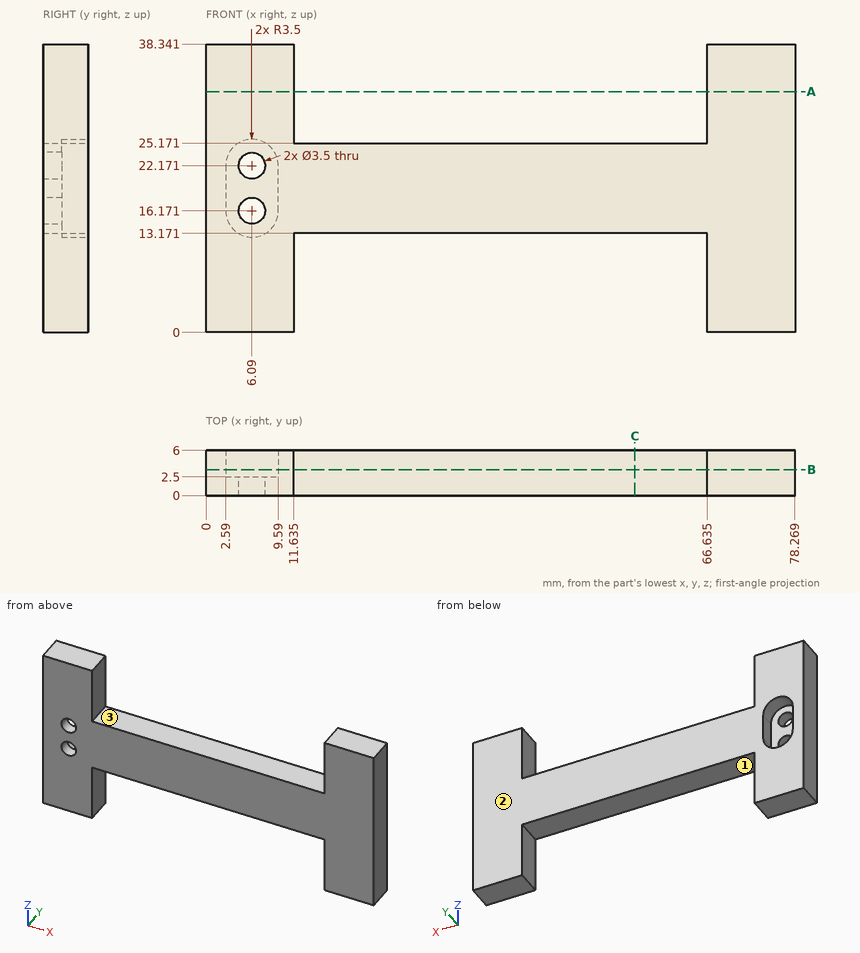
Print and shaded views of the part. All mm, measured from the part's lowest x, y and z. A direction names the side the tool comes from. Coordinates: 2 decimals unless noted, no trailing zeros. Order: outer loops, then holes, each group sorted by start corner. A loop starts at its lowest first (then second) coordinate and runs counter-clockwise, first axis right, second up. Notation, with made-up numbers: (74, -16) - (85, -16) arc R18 ccw to (85, 18) - close; hole circle Ø1 at (26, 29.25). An arc over 180 degrees is marked (long way). Return JSON: item names as keys, results as strings. Group by question number.
Item 1: Pin check, flat tips, straight feed: pin 1 (5.5 mm diameter, centred on x = 6.5, z = 17.5, fed in from +Y); pin 2 (3 mm diameter, centred on x = 45, y = 4.5, fed in from -Z). Stop position of each tip, or through.
Item 2: Cut at C-C (x = 57). List the corners of the cut face in (y, z), plus the area to 3 significant figures.
Item 3: Cut at B-B (y = 3.45). List the corners of the cut face in (x, z) (1 decimal), plus the area to 3 significant figures.
Item 4: Drill centre lines: probe 1 along X at (y, z) = (4.05, 10) (1 decimal); probe 2 along X at (y, z) = (5.3, 21.5); probe 3 along Z at (x, y) = (58, 0.4). Where is each one in solid material? Low to high. Write a range as from..to.
Item 5: Cut at A-A (z = 32). List the corners of the cut face in (x, y) (1 decimal), plus the area to 3 significant figures.
Item 6: Which spindle directions (+Z, -Z, +X, -X, +Y, -Y) get a long thin tool onto all of the face, cutting with end or side? Do the marked faces 1, 2 and 3. Say none if no direction does.
Check values:
{
 "1": {"pin 1": "stops at y = 2.5", "pin 2": "stops at z = 13.17"},
 "2": {"outline": "(0, 13.17) - (6, 13.17) - (6, 25.17) - (0, 25.17) - close", "area": "72.0 mm2"},
 "3": {"outline": "(0, 0) - (11.6, 0) - (11.6, 13.2) - (66.6, 13.2) - (66.6, 0) - (78.3, 0) - (78.3, 38.3) - (66.6, 38.3) - (66.6, 25.2) - (11.6, 25.2) - (11.6, 38.3) - (0, 38.3) - close; hole (2.6, 16.2) arc R3.5 ccw to (9.6, 16.2) - (9.6, 22.2) arc R3.5 ccw to (2.6, 22.2) - close", "area": "1,470 mm2"},
 "4": {"probe 1": "x = 0..11.6, 66.6..78.3", "probe 2": "x = 0..2.59, 9.59..78.27", "probe 3": "z = 13.17..25.17"},
 "5": {"outline": "(0, 0) - (11.6, 0) - (11.6, 6) - (0, 6) - close; (66.6, 0) - (78.3, 0) - (78.3, 6) - (66.6, 6) - close", "area": "140 mm2"},
 "6": {"face 1": "-Z, +Y, -Y", "face 2": "+Z, -Z, +X, -X, +Y", "face 3": "+Z, +Y, -Y"}
}
